```python
from build123d import *

# Parameters (mm, degrees)
F1_DEPTH = 50
F2_R     = 30
F4_DEPTH = 9.585521368
F5_R     = 5


with BuildPart() as f1:
    # F0 (on Top) → F1 (new body)
    with BuildSketch(Plane.XY):
        with BuildLine():
            ThreePointArc((75, 0), (0, -6.585521268), (-75, 0))
            Line((-75, 0), (-75.3485405324, -1.9693957188))
            ThreePointArc((-75.3485405324, -1.9693957188), (0, -8.585521268), (75.3485405324, -1.9693957188))
            Line((75.3485405324, -1.9693957188), (75, 0))
        make_face()
    extrude(amount=F1_DEPTH)

    # F2
    f2_edges = [f1.edges().sort_by_distance(p)[0] for p in [
        (75.17427, -0.984698, 0),
        (-75.17427, -0.984698, 0),
    ]]
    fillet(f2_edges, radius=F2_R)

    # F3 (on Front) → F4 (cut, up to face)
    with BuildSketch(Plane.XZ):
        with BuildLine():
            Line((-20, 0), (0, 0))
            Line((0, 0), (20, 0))
            add(Edge.make_bspline(
                [(20, 0), (18.7029346188, 4.7944349411), (15.9903043356, 14.8213230228), (5.4831015914, 20.0955088265), (0, 22.8478014469)],
                knots=[0, 0, 0, 0, 0.4781578195, 1, 1, 1, 1], degree=3))
            add(Edge.make_bspline(
                [(-20, 0), (-18.7029346188, 4.7944349411), (-15.9903043356, 14.8213230228), (-5.4831015914, 20.0955088265), (0, 22.8478014469)],
                knots=[0, 0, 0, 0, 0.4781578195, 1, 1, 1, 1], degree=3))
        make_face()
    extrude(amount=F4_DEPTH, mode=Mode.SUBTRACT)

    # F5
    f5_edges = [f1.edges().sort_by_distance(p)[0] for p in [
        (0, -7.585521, 22.847801),
    ]]
    fillet(f5_edges, radius=F5_R)


solid = f1.part
```
Can you work these out from the model? Positions are in its coordinate system, mm. Give positions to 0.01 mm unless a question says otherwise; leave off trailing zeros. Order: outer loops, then holes, each group sorted by start corner. A loop starts at its lowest first (then second) coordinate and runs counter-clockwise, first axis right, second up. Notation, with made-up numbers: M 47.25,76 L 86.25,76 A15 ccw 86.25,98 Z; hole C -20.75,86 d5. An arc over 180 degrees is marked long. Write item = value, one per line. Start each with the question number.
Q1. I need wall thicknesses on probe 1 along Y at (x, z) = (30, 14); probe 2 along Y at (x, z) = (-52, 13); probe 3 along Z at (x, y) = (-10.5, -6.5). Which ranges of each line are inside material? Lowest first, please. Write a range as [from, to].
Q2. Will these pins go through, and if not, where does the flat tip stop? pin 1 Ø2 at (x, z) = (-17.5, 30) entering from +Y; pin 2 Ø10 at (x, z) = (-26, 30.5) entering from +Y; pin 3 Ø2 at (x, z) = (-41, 32.5) entering from +Y.
Q3. Suppose I cut it at A-A (z = 36). Write out the boundary of the cut face in (x, y), plus the area to 3 significant figures.
Q4. Suppose I cut it at B-B (x = 36.5). Write out the boundary of the cut face in (y, z), plus the area to 3 significant figures.
Check result:
q1.probe_1 = [-7.54, -5.54]
q1.probe_2 = [-5.45, -3.43]
q1.probe_3 = [16.84, 50]
q2.pin_1 = -6.19
q2.pin_2 = -5.47
q2.pin_3 = -4.53
q3.outline = M -75.35,-1.97 A432.37 ccw 75.35,-1.97 L 75,0 A430.37 cw -75,0 Z
q3.area = 302 mm2
q4.outline = M -7.04,0 L -5.03,0 L -5.03,50 L -7.04,50 Z
q4.area = 100 mm2
